Read the model definition and answer for the solid it produces. Units are mm, in the model's axes. Face numbers are marked on the shaded views. A direction names the side the tool comes from. Coordinates: 2 decimals unless noted, no trailing zeros. Loops run counter-clockwise (first coordinate to the right, second up) from the corner with the lowest first, then second, coordinate; pieces in that order, holes last. Notation, with made-up numbers: M 51,71.25 L 90,71.25 A22 cw 90,77.25 Z; hole C -21.5,-32 d4. An arc over 180 degrees is marked long. One line per item, written item: value. Start each with the question number.
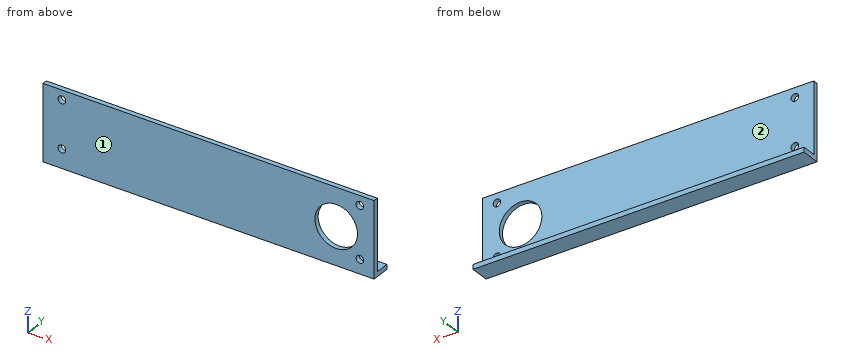
Autodesk Inventor part; units mm, degrees
ref_plane "YZ Plane" through (0, 0, 0) normal (1, 0, 0) x (0, 1, 0)
ref_plane "XZ Plane" through (0, 0, 0) normal (0, 1, 0) x (-1, 0, 0)
ref_plane "XY Plane" through (0, 0, 0) normal (0, 0, 1) x (1, 0, 0)
sketch "Sketch1" plane through (0, 0, 0) normal (0, 0, 1) x (1, 0, 0)
  line L0 (0, 0) -> (222.25, 0)
  line L1 (0, 0) -> (0, 3.175)
  line L2 (0, 3.175) -> (222.25, 3.175)
  line L3 (0, 3.175) -> (0, 12.7)
  line L4 (0, 12.7) -> (222.25, 12.7)
  line L5 (222.25, 0) -> (222.25, 12.7)
  dimension "d4" = 3.175
  dimension "d9" = 12.7
  dimension "d11" = 222.25
extrude "Extrusion1" add sketch "Sketch1" along normal blind 3.175
extrude "Extrusion2" add sketch "Sketch1" along normal blind 50.8 contours L1 L2 L5 L0
sketch "Sketch2" plane through (0, 0, 0) normal (0, -1, 0) x (1, 0, 0)
  circle A0 centre (196.85, 25.4) radius 14.2875
  line L0 (0, 0) -> (0, 50.8)
  line L1 (0, 0) -> (222.25, 0)
  line L2 (222.25, 0) -> (222.25, 50.8)
  line L3 (222.25, 50.8) -> (0, 50.8)
  circle A1 centre (12.7, 44.45) radius 2.54
  circle A2 centre (12.7, 12.7) radius 2.54
  circle A3 centre (212.725, 44.45) radius 2.54
  circle A4 centre (212.725, 9.525) radius 2.54
  dimension "d26" = 25.4
  dimension "d27" = 25.4
  dimension "d28" = 28.575
  dimension "d29" = 5.08
  dimension "d30" = 12.7
  dimension "d31" = 6.35
  dimension "d32" = 12.7
  dimension "d33" = 12.7
  dimension "d34" = 6.35
  dimension "d35" = 9.525
  dimension "d36" = 9.525
  dimension "d37" = 9.525
extrude "Extrusion3" cut sketch "Sketch2" against normal through all contours A0 | A1 | A2 | A3 | A4
equation "\"d4\" = d6"
equation "\"d30\" = d32"
equation "\"d34\" = d31"
equation "\"d36\" = d35"
properties part number "8 ball bottom 1 by 2 L short"
1) Flat-ended cylindrical pins translate along their axes: pin 1 (8 mm diameter, centred on x = 168, z = 43.5, fed in from +Y) (3 decimals); pin 2 (3 mm diameter, centred on x = 148.5, y = 8, fed in from +Z) (3 decimals). Find the tip coordinate at first contact, or state that the pin passes through.
2) Consider line 1 along Z through (x, y) = (12.7, 2); line 2 along Y through (x, z) = (24.5, 16) (3 decimals). Determine where each line is inside the solid, lowest interval first.
3) A tool of negligible diameter and unlimited length cuts with its end or side. For the marked faces 1 and 2, from which of +Z, -Z, +X, -X, +Y, -Y can it reach the whole face along a straight path? Write none if from no direction.
4) Section D-D (y = 9) is taken. Determine the outline of the cut face in (x, z) (3 decimals), then the cut area to 3 significant figures.
5) Section B-B (z = 44.45) is taken. Determine the outline of the cut face in (x, y) (3 decimals).
6) Section C-C (x = 196.85) is taken. Determine the outline of the cut face in (y, z) (1 decimal), then the cut area to 3 significant figures.
Results found:
1. pin 1: stops at y = 3.175
1. pin 2: stops at z = 3.175
2. line 1: z = 0 to 10.16, 15.24 to 41.91, 46.99 to 50.8
2. line 2: y = 0 to 3.175
3. face 1: +Z, -Z, +X, -X, -Y
3. face 2: +Z, +X, -X, +Y
4. outline: M 0,0 L 222.25,0 L 222.25,3.175 L 0,3.175 Z
4. area: 706 mm²
5. outline: M 0,0 L 10.16,0 L 10.16,3.175 L 0,3.175 Z; M 15.24,0 L 210.185,0 L 210.185,3.175 L 15.24,3.175 Z; M 215.265,0 L 222.25,0 L 222.25,3.175 L 215.265,3.175 Z
6. outline: M 0,0 L 12.7,0 L 12.7,3.2 L 3.2,3.2 L 3.2,11.1 L 0,11.1 Z; M 0,39.7 L 3.2,39.7 L 3.2,50.8 L 0,50.8 Z
6. area: 101 mm²
